from build123d import *

# Parameters (mm, degrees)
SKELETON_W          = 134
SKELETON_H          = 158
SKELETON_R          = 1.35
BOSS_EXTRUDE1_DEPTH = 4
BOSS_EXTRUDE2_START = -85
BOSS_EXTRUDE2_DEPTH = 85


with BuildPart() as part:
    # SKELETON → Boss-Extrude1 (new body)
    with BuildSketch(Plane.XY):
        with Locations((67, 75)):
            Rectangle(SKELETON_W, SKELETON_H)
        with Locations((28.381789687, 76.742237148)):
            Circle(SKELETON_R, mode=Mode.SUBTRACT)
        with Locations((10.500607165, 96.922428852)):
            Circle(SKELETON_R, mode=Mode.SUBTRACT)
        with Locations((126.445833013, 81.02799961)):
            Circle(SKELETON_R, mode=Mode.SUBTRACT)
        with Locations((34.46465583, 13.502410031)):
            Circle(SKELETON_R, mode=Mode.SUBTRACT)
        with Locations((117.09085583, 61.838610031)):
            Circle(SKELETON_R, mode=Mode.SUBTRACT)
    extrude(amount=BOSS_EXTRUDE1_DEPTH)

    # SKELETON<3> → Boss-Extrude2 (add)
    with BuildSketch(Plane.XY.offset(BOSS_EXTRUDE2_START)):
        Polygon((134, 154), (0, 154), (0, 150), (130, 150), (130, 0), (0, 0), (0, -4), (134, -4), align=None)
    extrude(amount=BOSS_EXTRUDE2_DEPTH)


solid = part.part
Geometry check sheet. Reference: the model listing, model coordinates, mm. A direction names the side the tool comes from. Give positions to 0.01 mm unless a question says otherwise; leave off trailing zeros. Order: outer loops, then holes, each group sorted by start corner. A loop starts at its lowest first (then second) coordinate and runs counter-clockwise, first axis right, second up.
1. Sectioned sample at C-C (x = 72.5). Record the boundary of the cut face in (y, z), then the cut area to 3 significant figures.
Completed:
outline: (-4, -85) - (0, -85) - (0, 0) - (150, 0) - (150, -85) - (154, -85) - (154, 4) - (-4, 4) - close
area: 1,310 mm2
2. Access from +Z, -Z, +X, -X, +Y, -Y to the whole of each face (thin tool, end or side, straight path). Record for faces 5 (the face through (66, -4, -41)), 6 (the face through (66, 0, -43)).
Completed:
face 5: +Z, -Z, +X, -X, -Y
face 6: -Z, -X
3. Sectioned sample at A-A (z = -6). Record the boundary of the cut face in (x, y).
Completed:
outline: (0, -4) - (134, -4) - (134, 154) - (0, 154) - (0, 150) - (130, 150) - (130, 0) - (0, 0) - close
4. Sectioned sample at B-B (y = 32.5). Record the boundary of the cut face in (x, z), then the cut area to 3 significant figures.
Completed:
outline: (0, 0) - (130, 0) - (130, -85) - (134, -85) - (134, 4) - (0, 4) - close
area: 876 mm2
5. Depth check by flat-ended pin: pin 1 (2.5 mm diameter, centred on x = 34.46, y = 13.5, fed in from -Z); pin 2 (4 mm diameter, centred on y = 113, z = -55, fed in from -X); pin 3 (12 mm diameter, centred on x = 110.5, y = 134.5, fed in from -Z); pin 4 (4.5 mm diameter, centred on x = 126.45, y = 81.03, fed in from +Z). Enter the tip coordinate at first touch or a pass-through.
Completed:
pin 1: passes through
pin 2: stops at x = 130
pin 3: stops at z = 0
pin 4: stops at z = 4
6. Scan lines: line 1 (Y direction, x = 70, z = -60); line 2 (Z direction, x = 6, y = 30); line 3 (X direction, y = 6.5, z = -31.5). Record each from-to range of solid material in increasing order.
Completed:
line 1: y = -4 to 0, 150 to 154
line 2: z = 0 to 4
line 3: x = 130 to 134
7. Draft check along Y on faces 1 (the face through (130, 76, -43)), 2 (the face through (64, 76, 0)), 3 (the face through (131, 75, -85)), 4 (the face through (68, 154, -41)). Enter one of: pulls with the +Y half, pulls with the -Y half, needs draft (parallel to the pull), parting line crosses it, or undercut.
Completed:
face 1: undercut
face 2: undercut
face 3: needs draft
face 4: pulls with the +Y half
